from build123d import *

# Parameters (mm, degrees)
SKETCH1_W           = 410
SKETCH1_H           = 120
BOSS_EXTRUDE1_DEPTH = 4
CUT_EXTRUDE1_REACH  = 215.638
SKETCH2_W           = 50.170218681
SKETCH2_H           = 70.735007755


with BuildPart() as part:
    # Sketch1 → Boss-Extrude1 (new body)
    with BuildSketch(Plane(origin=(0, 0, 0), x_dir=(1, 0, 0), z_dir=(0, 1, 0))):
        Rectangle(SKETCH1_W, SKETCH1_H)
    extrude(amount=BOSS_EXTRUDE1_DEPTH)

    # Sketch2 → Cut-Extrude1 (cut, up to next)
    with BuildSketch(Plane(origin=(0, 4, 0), x_dir=(1, 0, 0), z_dir=(0, 1, 0)), mode=Mode.PRIVATE) as cut_extrude1_sk1:
        with Locations((208.085109341, 45.367503877)):
            Rectangle(SKETCH2_W, SKETCH2_H)
    cut_extrude1_tool1 = extrude(cut_extrude1_sk1.sketch, amount=-CUT_EXTRUDE1_REACH, mode=Mode.PRIVATE) & part.part
    # Sketch2 → Cut-Extrude1 (cut, up to next)
    with BuildSketch(Plane(origin=(0, 4, 0), x_dir=(1, 0, 0), z_dir=(0, 1, 0)), mode=Mode.PRIVATE) as cut_extrude1_sk2:
        with Locations((-208.085109341, 45.367503877)):
            Rectangle(SKETCH2_W, SKETCH2_H)
    cut_extrude1_tool2 = extrude(cut_extrude1_sk2.sketch, amount=-CUT_EXTRUDE1_REACH, mode=Mode.PRIVATE) & part.part
    add(cut_extrude1_tool1.solids().sort_by_distance((208.085109, 4, -45.367504))[0], mode=Mode.SUBTRACT)
    add(cut_extrude1_tool2.solids().sort_by_distance((-208.085109, 4, -45.367504))[0], mode=Mode.SUBTRACT)


solid = part.part
Geometry: final body of the model. Coordinates: model frame, mm. Give positions to 0.01 mm unless a question says otherwise; leave off trailing zeros. Write each loop counter-clockwise with the first axis right and the second up, starting at its lowest first coordinate (ties: lowest second). Pieces come first, ordered by that corner, then holes. Notation, with made-up numbers: (58.25, -24.5) - (66.25, -24.5) arc R30 ccw to (66.25, 2.5) - close; hole circle Ø1 at (-29, 47.5). An arc over 180 degrees is marked (long way). Return JSON: item names as keys, results as strings. Group by question number.
1) Line query: line 1 (X direction, y = 2.65, z = -46). Output: solid intervals per line, ascending.
2) First-contact query: P1, Ø1.5, axis at y = 2.5, z = -15, coming from the -X side; P2, Ø1, axis at x = -101.5, z = -16.5, coming from the -Y side; P3, Ø1.2, axis at x = 197.5, y = 3, coming from the -Z side; P4, Ø2, axis at y = 2, z = -47.5, coming from the +X side. Flat tips, straight axial feed; report the tip coordinate or a pass-through.
3) Section A-A on y = 1.75. Return the cut outline in (x, z).
4) Section B-B on z = -49. Return the cut outline in (x, y), plus the area to 3 significant figures.
Filled in:
{
 "1": {"line 1": "x = -183 to 183"},
 "2": {"P1": "stops at x = -183", "P2": "stops at y = 0", "P3": "stops at z = -10", "P4": "stops at x = 183"},
 "3": {"outline": "(-205, -10) - (-183, -10) - (-183, -60) - (183, -60) - (183, -10) - (205, -10) - (205, 60) - (-205, 60) - close"},
 "4": {"outline": "(-183, 0) - (183, 0) - (183, 4) - (-183, 4) - close", "area": "1,460 mm^2"}
}
